Input: dimensioned drawing with shaded views. Units: mm. Origin: part minimum x, y, z. Round coordinates to 2 decimals unless told otherwise and drop trailing zeros. Order: outer loops, then holes, each group sorted by start corner. A loop starts at its lowest first (then second) coordinate and runs counter-clockwise, first axis right, second up.
Item 1: Cut plane C-C on z = 7.5. Output: boundary loops of the cut face in (x, y).
Item 2: First-contact query: pin 1 (8 mm diameter, centred on x = 15, y = 15, fed in from +Z); pin 2 (8 mm diameter, centred on x = 13, y = 14, fed in from +Z); pin 3 (4 mm diameter, centred on x = 12, z = 15.5, fed in from -Y); pin 4 (1 mm diameter, centred on x = 14.5, z = 40.5, fed in from -Y). Flat tips, straight axial feed; report the tip coordinate or a pass-through.
Item 3: Cut plane B-B on z = 40. Output: boundary loops of the cut face in (x, y), then the cut area to 3 significant figures.
Item 4: Line query: L1, parallel to Y at x = 10.5, z = 9; L2, parallel to Y at x = 15, z = 1; L3, parallel to X at y = 16, z = 19. Output: solid intervals per line, ascending.
Item 5: Mould query, pull axis X, two halves, no side actions, for the marked faces 1, 2 and 3. Classes: released by +X, released by -X, zero draft, split by the parting line, or undercut.
Item 6: Cut plane A-A on x = 15. Output: boundary loops of the cut face in (y, z).
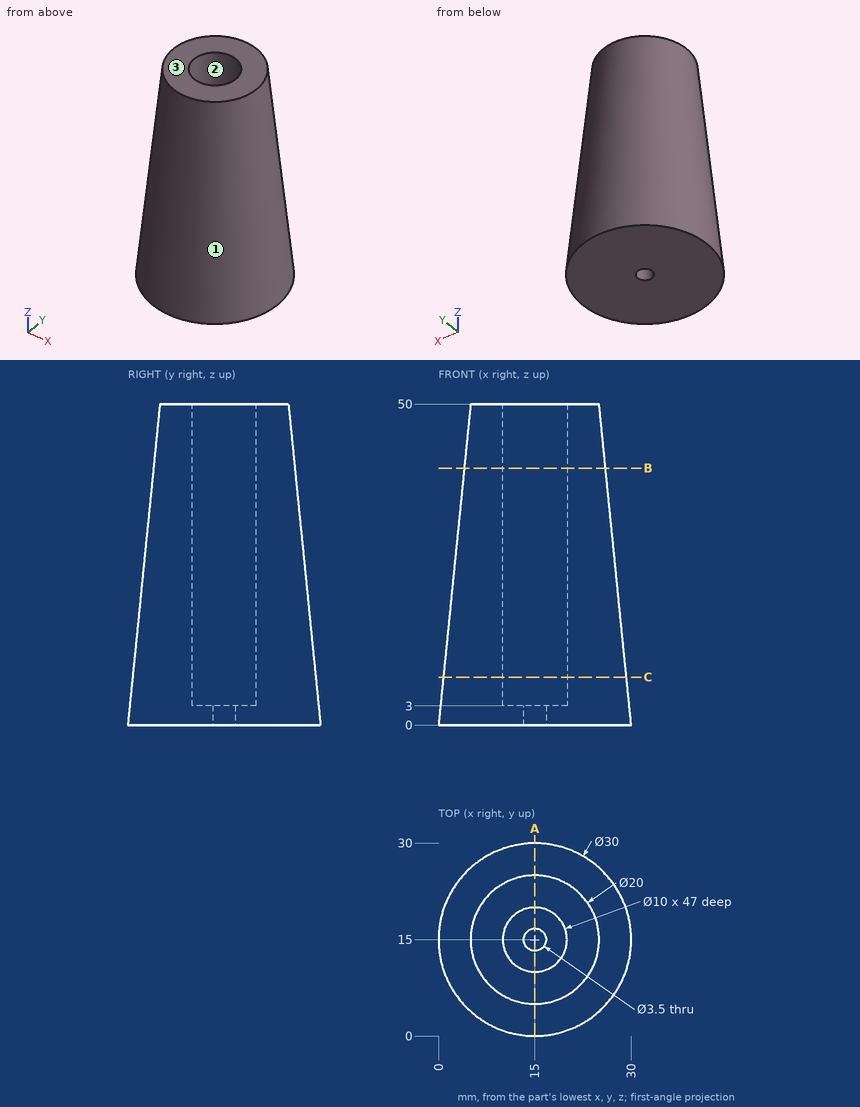
From the geometry:
1. outline: circle Ø28.5 at (15, 15); hole circle Ø10 at (15, 15)
2. pin 1: stops at z = 3
2. pin 2: stops at z = 50
2. pin 3: stops at y = 1.5
2. pin 4: stops at y = 4.01
3. outline: circle Ø22 at (15, 15); hole circle Ø10 at (15, 15)
3. area: 302 mm2
4. L1: y = 1.64 to 12.82, 17.18 to 28.36
4. L2: y = 0.1 to 13.25, 16.75 to 29.9
4. L3: x = 1.94 to 10.1, 19.9 to 28.06
5. face 1: split by the parting line
5. face 2: undercut
5. face 3: zero draft
6. outline: (0, 0) - (13.25, 0) - (13.25, 3) - (10, 3) - (10, 50) - (5, 50) - close; (16.75, 0) - (30, 0) - (25, 50) - (20, 50) - (20, 3) - (16.75, 3) - close
